Here's how the part is built. I have some questions about the finished solid (model axes, mm). A direction names the side the tool comes from. Give positions to 0.01 mm unless a question says otherwise; leave off trailing zeros. Write each loop counter-clockwise with the first axis right and the second up, starting at its lowest first coordinate (ties: lowest second). Pieces come first, ordered by that corner, then holes. Notation, with made-up numbers: (74, 50.25) - (100, 50.25) arc R22 ccw to (100, 87.25) - close; hole circle Ø11 at (64, 49.5). An arc over 180 degrees is marked (long way). Use a Markdown table: item, result.
```python
from build123d import *

# Parameters (mm, degrees)
ESQUISSE1_R             = 22.5
BOSS_EXTRU_1_DEPTH      = 60
ESQUISSE2_OUTSIDE_W     = 64.492
ESQUISSE2_OUTSIDE_H     = 64.492
ESQUISSE2_OUTSIDE_R     = 17.5
ENL_V_MAT_EXTRU_1_DEPTH = 27
ESQUISSE3_OUTSIDE_W     = 64.492
ESQUISSE3_OUTSIDE_H     = 64.492
ESQUISSE3_OUTSIDE_R     = 17.5
ENL_V_MAT_EXTRU_2_DEPTH = 21.5
ESQUISSE4_R             = 12.5
ENL_V_MAT_EXTRU_3_DEPTH = 61
ENL_V_MAT_EXTRU_4_DEPTH = 15.8
CHANFREIN1_SIZE         = 1


with BuildPart() as part:
    # Esquisse1 → Boss.-Extru.1 (new body)
    with BuildSketch(Plane.XY):
        Circle(ESQUISSE1_R)
    extrude(amount=BOSS_EXTRU_1_DEPTH)

    # Esquisse2 outside → Enlèv. mat.-Extru.1 (cut)
    with BuildSketch(Plane.XY.offset(60)):
        Rectangle(ESQUISSE2_OUTSIDE_W, ESQUISSE2_OUTSIDE_H)
        Circle(ESQUISSE2_OUTSIDE_R, mode=Mode.SUBTRACT)
    extrude(amount=-ENL_V_MAT_EXTRU_1_DEPTH, mode=Mode.SUBTRACT)

    # Esquisse3 outside → Enlèv. mat.-Extru.2 (cut)
    with BuildSketch(Plane(origin=(0, 0, 0), x_dir=(-1, 0, 0), z_dir=(0, 0, -1))):
        Rectangle(ESQUISSE3_OUTSIDE_W, ESQUISSE3_OUTSIDE_H)
        with Locations(Location((0, 0, 0), (0, 0, 180))):  # turned: the seam where the file's is
            Circle(ESQUISSE3_OUTSIDE_R, mode=Mode.SUBTRACT)
    extrude(amount=-ENL_V_MAT_EXTRU_2_DEPTH, mode=Mode.SUBTRACT)

    # Esquisse4 → Enlèv. mat.-Extru.3 (cut, through all)
    with BuildSketch(Plane.XY.offset(60)):
        Circle(ESQUISSE4_R)
    extrude(amount=-ENL_V_MAT_EXTRU_3_DEPTH, mode=Mode.SUBTRACT)

    # Esquisse6 → Enlèv. mat.-Extru.4 (cut)
    with BuildSketch(Plane(origin=(0, 0, 0), x_dir=(1, 0, 0), z_dir=(0, 1, 0))):
        with BuildLine():
            Line((-3.5, -132.654252639), (-3.5, 6.73879401))
            ThreePointArc((-3.5, 6.73879401), (0, 10.23879401), (3.5, 6.73879401))
            Line((3.5, 6.73879401), (3.5, -132.654252639))
            ThreePointArc((3.5, -132.654252639), (0, -136.154252639), (-3.5, -132.654252639))
        make_face()
    extrude(amount=-ENL_V_MAT_EXTRU_4_DEPTH, mode=Mode.SUBTRACT)

    # Chanfrein1
    chanfrein1_edges = [part.edges().sort_by_distance(p)[0] for p in [
        (-17.5, 0, 60),
    ]]
    chamfer(chanfrein1_edges, length=CHANFREIN1_SIZE)


solid = part.part
```
Item 1: I need wall thicknesses on line 1 along Y through (x, z) = (0, 26); line 2 along Y through (x, z) = (0, 44); line 3 along Z through (x, y) = (-6, -18). Which ranges of each line are inside material? Lowest first, please. Write a range as [from, to].
Values:
| item | result |
|---|---|
| line 1 | y = [-22.5, -15.8], [12.5, 22.5] |
| line 2 | y = [-17.5, -15.8], [12.5, 17.5] |
| line 3 | z = [21.5, 33] |
Item 2: If we section it at C-C, the plane z = 26: Write out the boundary of the cut face in (x, y).
Values:
| item | result |
|---|---|
| outline | circle Ø45 at (0, 0); hole (-3.5, -15.8) - (3.5, -15.8) - (3.5, -12) arc R12.5 ccw (long way) to (-3.5, -12) - close |
Item 3: Will these pins go through, and if not, where does the flat tip stop? pin 1 Ø5.5 at (x, z) = (-1, 33.5) entering from +Y; pin 2 Ø8 at (y, z) = (-5, 32.5) entering from +X; pin 3 Ø4 at (y, z) = (-18, 40) entering from -X; pin 4 Ø13.5 at (x, y) = (2.5, 0.5) entering from +Z.
Values:
| item | result |
|---|---|
| pin 1 | stops at y = 22.5 |
| pin 2 | stops at x = 22.48 |
| pin 3 | stops at x = -7.09 |
| pin 4 | passes through |
Item 4: Thinking about a two-plate mould opening in Y: for faces 4 (the flat face through (12, -13, 33)), 5 (the flat face through (0, -15.8, 30)), 6 (the cylindrical face through (-13.887, -10.648, 46.182)), which applies, +Y half, -Y half, draft (parallel to the pull), parting line (faces both ways), or undercut?
Values:
| item | result |
|---|---|
| face 4 | draft |
| face 5 | undercut |
| face 6 | parting line |
Item 5: If we section it at A-A, the plane x = 0: Write out the boundary of the cut face in (y, z).
Values:
| item | result |
|---|---|
| outline | (-22.5, 21.5) - (-17.5, 21.5) - (-17.5, 0) - (-15.8, 0) - (-15.8, 60) - (-16.5, 60) - (-17.5, 59) - (-17.5, 33) - (-22.5, 33) - close; (12.5, 0) - (17.5, 0) - (17.5, 21.5) - (22.5, 21.5) - (22.5, 33) - (17.5, 33) - (17.5, 59) - (16.5, 60) - (12.5, 60) - close |
Item 6: If we section it at D-D, the plane z = 40.5: Write out the boundary of the cut face in (x, y).
Values:
| item | result |
|---|---|
| outline | circle Ø35 at (0, 0); hole (-3.5, -15.8) - (3.5, -15.8) - (3.5, -12) arc R12.5 ccw (long way) to (-3.5, -12) - close |
Item 7: For faces 1 (the flat face through (-12, -13, 21.5)), 2 (the flat face through (-3.5, -14, 30)), 3 (the flat face through (-5, 12, 0)), which set-ups out of +Z, -Z, +X, -X, +Y, -Y let a thin tool reach every point of the face, with its end or its side?
Values:
| item | result |
|---|---|
| face 1 | -Z |
| face 2 | +Z, -Z |
| face 3 | -Z, +X, -X, +Y, -Y |
Item 8: If we section it at B-B, the plane y = 0: Write out the boundary of the cut face in (x, z).
Values:
| item | result |
|---|---|
| outline | (-22.5, 21.5) - (-17.5, 21.5) - (-17.5, 0) - (-12.5, 0) - (-12.5, 60) - (-16.5, 60) - (-17.5, 59) - (-17.5, 33) - (-22.5, 33) - close; (12.5, 0) - (17.5, 0) - (17.5, 21.5) - (22.5, 21.5) - (22.5, 33) - (17.5, 33) - (17.5, 59) - (16.5, 60) - (12.5, 60) - close |
